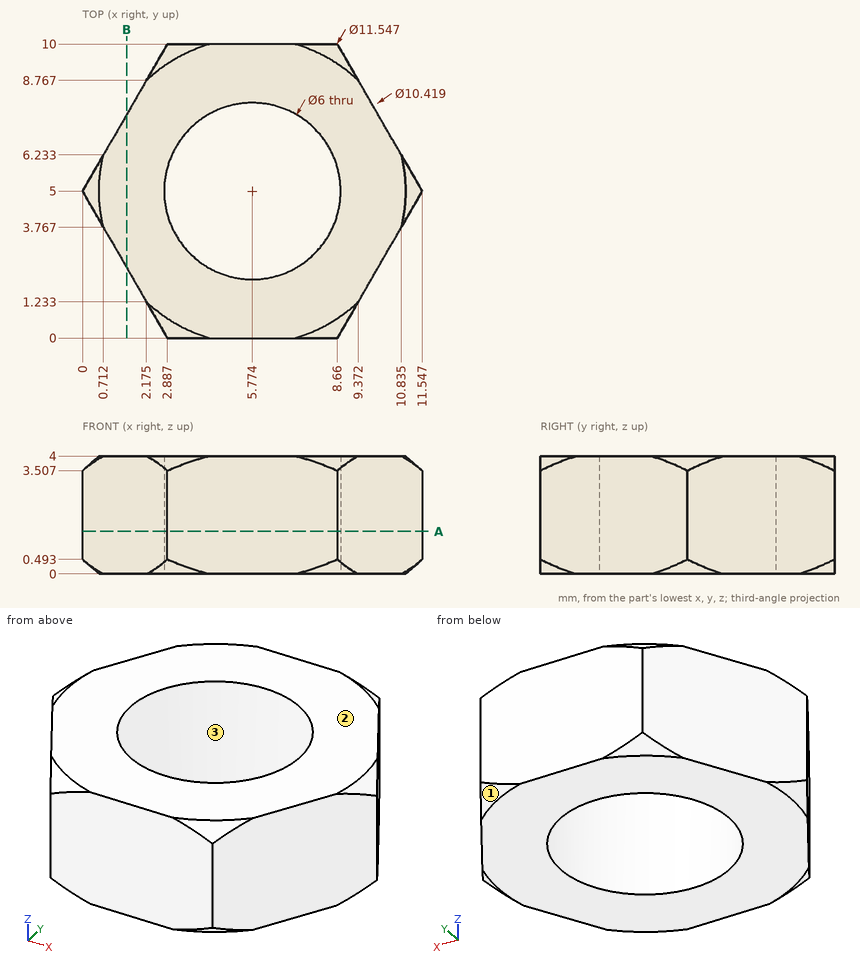
Check sheet for the drawn part. Datum: minimum x, y, z corner. Units: mm. Coordinates: 2 decimals unless noted, no trailing zeros. Loops run counter-clockwise (first coordinate to the right, second up) from the corner with the lowest first, then second, coordinate; pieces in that order, holes last. Notation, with made-up numbers: M 54.5,18 L 84.5,18 A25 ccw 84.5,42 Z; hole C -38.75,-23 d3. An arc over 180 degrees is marked long. Answer as a JSON object with one key per item and string values.
1. Sectioned sample at B-B on x = 1.5. Record the cut outline in (y, z).
Outcome:
{"outline": "M 2.4,0 L 7.6,0 L 7.6,4 L 2.4,4 Z"}
2. Release check for a two-part mould opening along Y. For the marked faces 1, 2 and 3 record: pulls with the +Y half, pulls with the -Y half, needs draft (parallel to the pull), parting line crosses it, or undercut.
Outcome:
{"face 1": "pulls with the +Y half", "face 2": "needs draft", "face 3": "undercut"}
3. Scan lines: L1, parallel to Y at x = 8, z = 2.85; L2, parallel to Y at x = 5, z = 0.3; L3, parallel to Y at x = 10.5, z = 1.45 (1 decimal). Record each from-to range of solid material in increasing order. Write a range as from..to.
Outcome:
{"L1": "0..2.99, 7.01..10", "L2": "0..2.1, 7.9..10", "L3": "3.2..6.8"}
4. Sectioned sample at A-A on z = 1.45. Record the cut outline in (x, y).
Outcome:
{"outline": "M 0,5 L 2.89,0 L 8.66,0 L 11.55,5 L 8.66,10 L 2.89,10 Z; hole C 5.77,5 d6"}
5. Depth check by flat-ended pin: P1, Ø3.5, axis at x = 5.77, y = 5, coming from the +Z side. Enter the tip coordinate at first touch or a pass-through.
Outcome:
{"P1": "through"}
